CAD build for the part. Positions are in the model's coordinates, mm. Round coordinates to 2 decimals unless told otherwise and drop trailing zeros. Order: outer loops, then holes, each group sorted by start corner. A loop starts at its lowest first (then second) coordinate and runs counter-clockwise, first axis right, second up. Notation, with made-up numbers: M -14.75,83.25 L 13.25,83.25 A16 ccw 13.25,100.25 Z; hole C -16.5,-31 d3. An arc over 180 degrees is marked long. Put each result on its own line as item: value.
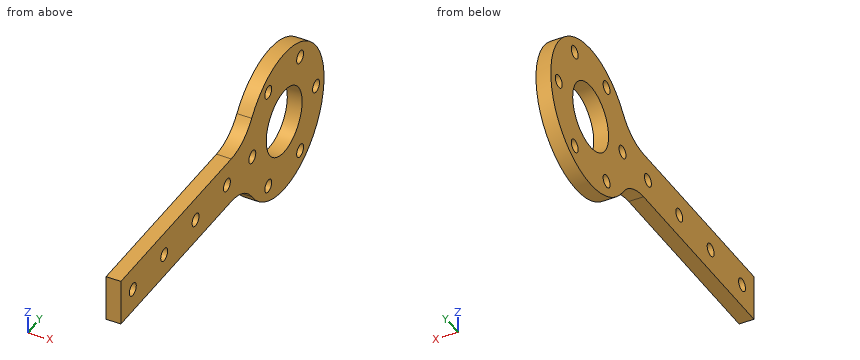
```python
from build123d import *

# Parameters (mm, degrees)
BOSS_EXTRUDE1_DEPTH = 6.35
FILLET1_R           = 20
SKETCH2_R           = 14.3
SKETCH2_R_2         = 2.75
CUT_EXTRUDE1_DEPTH  = 7.35
SKETCH3_R           = 2.75
CUT_EXTRUDE2_DEPTH  = 7.35


with BuildPart() as part:
    # Sketch1 → Boss-Extrude1 (new body)
    with BuildSketch(Plane(origin=(0, 0, 0), x_dir=(0, 0, -1), z_dir=(1, 0, 0))):
        with BuildLine():
            Line((-10, -30.134075396), (-10, -130.134075396))
            Line((-10, -130.134075396), (10, -130.134075396))
            Line((10, -130.134075396), (10, -30.134075396))
            ThreePointArc((10, -30.134075396), (0, 31.75), (-10, -30.134075396))
        make_face()
    extrude(amount=BOSS_EXTRUDE1_DEPTH)

    # Fillet1
    fillet1_edges = [part.edges().sort_by_distance(p)[0] for p in [
        (3.175, -30.134075396, -10),
        (3.175, -30.134075396, 10),
    ]]
    fillet(fillet1_edges, radius=FILLET1_R)

    # Sketch2 → Cut-Extrude1 (cut, through all)
    with BuildSketch(Plane(origin=(6.35, 0, 0), x_dir=(0, 0, -1), z_dir=(1, 0, 0))):
        Circle(SKETCH2_R)
        with Locations((0, 25.4)):
            Circle(SKETCH2_R_2)
        with Locations((21.997045256, 12.7)):
            Circle(SKETCH2_R_2)
        with Locations((21.997045256, -12.7)):
            Circle(SKETCH2_R_2)
        with Locations((0, -25.4)):
            Circle(SKETCH2_R_2)
        with Locations((-21.997045256, -12.7)):
            Circle(SKETCH2_R_2)
        with Locations((-21.997045256, 12.7)):
            Circle(SKETCH2_R_2)
    extrude(amount=-CUT_EXTRUDE1_DEPTH, mode=Mode.SUBTRACT)

    # Sketch3 → Cut-Extrude2 (cut, through all)
    with BuildSketch(Plane(origin=(6.35, 0, 0), x_dir=(0, 0, -1), z_dir=(1, 0, 0))):
        with Locations((0, -120.63662428)):
            Circle(SKETCH3_R)
        with Locations((0, -95.63662428)):
            Circle(SKETCH3_R)
        with Locations((0, -70.63662428)):
            Circle(SKETCH3_R)
        with Locations((0, -45.63662428)):
            Circle(SKETCH3_R)
    extrude(amount=-CUT_EXTRUDE2_DEPTH, mode=Mode.SUBTRACT)


solid = part.part
```
Item 1: Probe line 1 along Z through (x, y) = (3.75, -46); line 2 along Z through (x, y) = (5.25, -100.5); line 3 along Y through (x, z) = (2, -8.5). List the from-to ranges inside material, lowest first. Write a range as [from, to].
Answers below:
line 1: [-10, -2.73], [2.73, 10]
line 2: [-10, 10]
line 3: [-130.13, -11.5], [11.5, 30.59]
Item 2: Band-saw the part on B-B on z = 0. State how many separate pieces and enclosed holes the cut face has, and give its area (3 significant figures).
Answers below:
separate pieces: 8
enclosed holes: 0
area: 637 mm²
Item 3: Band-saw the part on A-A on y = 0. Give the cut face in (x, z).
Answers below:
outline: M 0,-31.75 L 6.35,-31.75 L 6.35,-14.3 L 0,-14.3 Z; M 0,14.3 L 6.35,14.3 L 6.35,31.75 L 0,31.75 Z
Item 4: Pin check, flat tips, straight feed: P1, Ø1.9, axis at x = 2, y = -82, coming from the -Z side; P2, Ø3, axis at x = 5, y = -3.5, coming from the -Z side; P3, Ø1.5, axis at x = 3, y = -57.5, coming from the +Z side. Stop position of each tip, or through.
Answers below:
P1: z = -10
P2: z = -31.69
P3: z = 10
Item 5: Band-saw the part on C-C on z = -22.5. Give the cut face in (x, y).
Answers below:
outline: M 0,-22.4 L 6.35,-22.4 L 6.35,-15.4 L 0,-15.4 Z; M 0,-10 L 6.35,-10 L 6.35,10 L 0,10 Z; M 0,15.4 L 6.35,15.4 L 6.35,22.4 L 0,22.4 Z
